Could you check a few things on this model? Use its own coordinates, in mm. A direction names the side the tool comes from. Round coordinates to 2 decimals unless told otherwise and drop trailing zeros. Write each loop counter-clockwise with the first axis right and the second up, starting at its lowest first coordinate (ties: lowest second). Pieces come first, ordered by that corner, then holes. Notation, with made-up numbers: (70, 83.5) -> (103, 83.5) arc R26 cw to (103, 105.5) -> close; hole circle Ø9 at (17, 41). An arc over 180 degrees is marked (long way). Return JSON: item names as keys, results as strings.
from build123d import *

# Parameters (mm, degrees)
EXTRUDE_1_DEPTH             = 20
CUT_EXTRUDE_1_DEPTH         = 15
EXTRUDE_2_DEPTH             = 15
HOLE_WIZARD_4_5_4_5_1_D     = 4.5
HOLE_WIZARD_4_5_4_5_1_DEPTH = 20
HOLE_WIZARD_20_0_20_1_D     = 20
HOLE_WIZARD_20_0_20_1_DEPTH = 20
HOLE_WIZARD_8_2_8_2_1_D     = 8.2
HOLE_WIZARD_8_2_8_2_1_DEPTH = 20
FILLET_1_R                  = 10


with BuildPart() as part:
    # 草图1 → 凸台-拉伸1 (new body)
    with BuildSketch(Plane(origin=(0, 0, 0), x_dir=(-1, 0, 0), z_dir=(0, 0, -1))):
        with BuildLine():
            ThreePointArc((-163.022889612, 198.274261736), (-150, 100), (-136.977110388, 198.274261736))
            ThreePointArc((-136.977110388, 198.274261736), (-140.459664046, 197.328853695), (-143.715646252, 195.773040012))
            ThreePointArc((-143.715646252, 195.773040012), (-144.596931613, 195.703918846), (-145.18869047, 196.36062508))
            ThreePointArc((-145.18869047, 196.36062508), (-150, 200), (-154.81130953, 196.36062508))
            ThreePointArc((-154.81130953, 196.36062508), (-155.403068387, 195.703918846), (-156.284353748, 195.773040012))
            ThreePointArc((-156.284353748, 195.773040012), (-159.540335954, 197.328853695), (-163.022889612, 198.274261736))
        make_face()
    extrude(amount=-EXTRUDE_1_DEPTH)

    # 草图2 → 切除-拉伸1 (cut)
    with BuildSketch(Plane.XY.offset(20)):
        with BuildLine():
            ThreePointArc((189.376148289, 164.838033327), (188.791059223, 165.557292987), (189.04835202, 166.448059))
            ThreePointArc((189.04835202, 166.448059), (189.837168574, 173), (183.768612947, 175.592835325))
            ThreePointArc((183.768612947, 175.592835325), (182.868540552, 175.815396233), (182.538187947, 176.681728058))
            ThreePointArc((182.538187947, 176.681728058), (169.336845119, 194.477731675), (150.795414997, 182.345602173))
            ThreePointArc((150.795414997, 182.345602173), (150.50949688, 181.851710417), (150, 181.594628396))
            ThreePointArc((150, 181.594628396), (149.49050312, 181.851710417), (149.204585003, 182.345602173))
            ThreePointArc((149.204585003, 182.345602173), (130.663154881, 194.477731675), (117.461812053, 176.681728058))
            ThreePointArc((117.461812053, 176.681728058), (117.131459448, 175.815396233), (116.231387053, 175.592835325))
            ThreePointArc((116.231387053, 175.592835325), (110.162831426, 173), (110.95164798, 166.448059))
            ThreePointArc((110.95164798, 166.448059), (111.208940777, 165.557292987), (110.623851711, 164.838033327))
            ThreePointArc((110.623851711, 164.838033327), (101.812731907, 144.507333265), (121.590179319, 134.516048507))
            ThreePointArc((121.590179319, 134.516048507), (122.160861185, 134.515382033), (122.638249186, 134.202685802))
            ThreePointArc((122.638249186, 134.202685802), (122.670358065, 133.63290755), (122.385594316, 133.138349319))
            ThreePointArc((122.385594316, 133.138349319), (121.149577026, 111.01493506), (143.162039659, 108.480238616))
            ThreePointArc((143.162039659, 108.480238616), (144.077481329, 108.62731078), (144.720260927, 107.959105675))
            ThreePointArc((144.720260927, 107.959105675), (150, 104), (155.279739073, 107.959105675))
            ThreePointArc((155.279739073, 107.959105675), (155.922518671, 108.62731078), (156.837960341, 108.480238616))
            ThreePointArc((156.837960341, 108.480238616), (178.850422974, 111.01493506), (177.614405684, 133.138349319))
            ThreePointArc((177.614405684, 133.138349319), (177.329641935, 133.63290755), (177.361750814, 134.202685802))
            ThreePointArc((177.361750814, 134.202685802), (177.839138815, 134.515382033), (178.409820681, 134.516048507))
            ThreePointArc((178.409820681, 134.516048507), (198.187268093, 144.507333265), (189.376148289, 164.838033327))
        make_face()
    extrude(amount=-CUT_EXTRUDE_1_DEPTH, mode=Mode.SUBTRACT)

    # 草图3 → 凸台-拉伸2 (add)
    with BuildSketch(Plane.XY.offset(5)):
        with BuildLine():
            ThreePointArc((150.795414997, 125.187925524), (150.50949688, 124.694033767), (150, 124.436951746))
            ThreePointArc((150, 124.436951746), (149.49050312, 124.694033767), (149.204585003, 125.187925524))
            ThreePointArc((149.204585003, 125.187925524), (141.575, 135.407471946), (128.909820681, 136.905113168))
            ThreePointArc((128.909820681, 136.905113168), (128.339138815, 136.905779642), (127.861750814, 137.218475873))
            ThreePointArc((127.861750814, 137.218475873), (127.829641935, 137.788254125), (128.114405684, 138.282812356))
            ThreePointArc((128.114405684, 138.282812356), (133.15, 150), (128.114405684, 161.717187644))
            ThreePointArc((128.114405684, 161.717187644), (127.829641935, 162.211745875), (127.861750814, 162.781524127))
            ThreePointArc((127.861750814, 162.781524127), (128.339138815, 163.094220358), (128.909820681, 163.094886832))
            ThreePointArc((128.909820681, 163.094886832), (141.575, 164.592528054), (149.204585003, 174.812074476))
            ThreePointArc((149.204585003, 174.812074476), (149.49050312, 175.305966233), (150, 175.563048254))
            ThreePointArc((150, 175.563048254), (150.50949688, 175.305966233), (150.795414997, 174.812074476))
            ThreePointArc((150.795414997, 174.812074476), (158.425, 164.592528054), (171.090179319, 163.094886832))
            ThreePointArc((171.090179319, 163.094886832), (171.660861185, 163.094220358), (172.138249186, 162.781524127))
            ThreePointArc((172.138249186, 162.781524127), (172.170358065, 162.211745875), (171.885594316, 161.717187644))
            ThreePointArc((171.885594316, 161.717187644), (166.85, 150), (171.885594316, 138.282812356))
            ThreePointArc((171.885594316, 138.282812356), (172.170358065, 137.788254125), (172.138249186, 137.218475873))
            ThreePointArc((172.138249186, 137.218475873), (171.660861185, 136.905779642), (171.090179319, 136.905113168))
            ThreePointArc((171.090179319, 136.905113168), (158.425, 135.407471946), (150.795414997, 125.187925524))
        make_face()
    extrude(amount=EXTRUDE_2_DEPTH)

    # Ø4.5 (4.5) 直径孔1
    with Locations(Plane(origin=(0, 0, 0), x_dir=(-1, 0, 0), z_dir=(0, 0, -1))):
        with Locations((-150, 195), (-111.02885683, 127.5), (-188.97114317, 127.5)):
            Hole(HOLE_WIZARD_4_5_4_5_1_D / 2, depth=HOLE_WIZARD_4_5_4_5_1_DEPTH)

    # Ø20.0 (20) 直径孔1
    with Locations(Plane(origin=(0, 0, 0), x_dir=(-1, 0, 0), z_dir=(0, 0, -1))):
        with Locations((-133.5, 178.578838325), (-117, 150), (-133.5, 121.421161675), (-166.5, 121.421161675), (-183, 150), (-166.5, 178.578838325)):
            Hole(HOLE_WIZARD_20_0_20_1_D / 2, depth=HOLE_WIZARD_20_0_20_1_DEPTH)

    # Ø8.2 (8.2) 直径孔1
    with Locations(Plane(origin=(0, 0, 0), x_dir=(-1, 0, 0), z_dir=(0, 0, -1))):
        with Locations((-114.925971147, 170.25), (-185.074028853, 170.25), (-150, 109.5)):
            Hole(HOLE_WIZARD_8_2_8_2_1_D / 2, depth=HOLE_WIZARD_8_2_8_2_1_DEPTH)

    # 圆角1
    fillet_1_edges = [part.edges().sort_by_distance(p)[0] for p in [
        (136.977110388, 198.274261736, 10),
        (163.022889612, 198.274261736, 10),
    ]]
    fillet(fillet_1_edges, radius=FILLET_1_R)


solid = part.part
1) I want a section at D-D, the plane x = 139.5. Count the separate pieces of the cut face and the enclosed holes in it, and give its area (3 significant figures).
Return value:
{"separate pieces": "3", "enclosed holes": "0", "area": "870 mm²"}
2) For faces 1 (the face through (151.97, 100.04, 9.86)), 2 (the face through (178.63, 110.76, 12.6)), 3 (the face through (157.68, 196.53, 9.86)), which set-ups out of +Z, -Z, +X, -X, +Y, -Y let a thin tool reach every point of the face, with its end or its side?
Return value:
{"face 1": "+Z, -Z", "face 2": "+Z", "face 3": "+Z, -Z, +Y"}
3) I want a section at A-A, the plane y = 154.5. Please give me the cut outline in (x, z).
Return value:
{"outline": "(100.2, 0) -> (108.07, 0) -> (108.07, 5) -> (101.49, 5) -> (101.49, 20) -> (100.2, 20) -> close; (125.93, 0) -> (174.07, 0) -> (174.07, 5) -> (167.49, 5) -> (167.49, 20) -> (132.51, 20) -> (132.51, 5) -> (125.93, 5) -> close; (191.93, 0) -> (199.8, 0) -> (199.8, 20) -> (198.51, 20) -> (198.51, 5) -> (191.93, 5) -> close"}
4) I want a section at C-C, the plane y = 190. Please give me the cut outline in (x, z).
Return value:
{"outline": "(120, 0) -> (180, 0) -> (180, 20) -> (177.92, 20) -> (177.92, 5) -> (155.08, 5) -> (155.08, 20) -> (144.92, 20) -> (144.92, 5) -> (122.08, 5) -> (122.08, 20) -> (120, 20) -> close"}
5) I want a section at B-B, the plane y = 127.5. Please give me the cut outline in (x, z).
Return value:
{"outline": "(105.35, 0) -> (108.78, 0) -> (108.78, 20) -> (105.35, 20) -> close; (113.28, 0) -> (125.56, 0) -> (125.56, 5) -> (118.54, 5) -> (118.54, 20) -> (113.28, 20) -> close; (141.44, 0) -> (158.56, 0) -> (158.56, 5) -> (151.54, 5) -> (151.54, 20) -> (148.46, 20) -> (148.46, 5) -> (141.44, 5) -> close; (174.44, 0) -> (186.72, 0) -> (186.72, 20) -> (181.46, 20) -> (181.46, 5) -> (174.44, 5) -> close; (191.22, 0) -> (194.65, 0) -> (194.65, 20) -> (191.22, 20) -> close"}
6) Will these pins go through, and if not, where does the flat tip stop? pin 1 Ø1 at (x, z) = (116.5, 4.5) entering from -Y; pin 2 Ø4 at (x, y) = (186.5, 162) entering from -Z; pin 3 Ø12 at (y, z) = (163, 9.5) entering from +X; pin 4 Ø4 at (x, y) = (188.97, 127.5) entering from -Z.
Return value:
{"pin 1": "y = 112.44", "pin 2": "z = 0", "pin 3": "x = 199.51", "pin 4": "through"}
7) Thinking about a two-plate mould opening in Y: for faces 4 (the face through (150, 184, 20)), 5 (the face through (117.13, 173.707, 2.535)), 6 (the face through (141.733, 135.315, 12.395)), 7 (the face through (142.28, 196.55, 9.86)), which applies, pulls with the +Y half, pulls with the -Y half, needs draft (parallel to the pull), parting line crosses it, or undercut?
Return value:
{"face 4": "needs draft", "face 5": "undercut", "face 6": "undercut", "face 7": "pulls with the +Y half"}
8) If I drill on probe 1 along X at (y, z) = (171, 4.5); probe 2 along Y at (x, z) = (189, 9); probe 3 along Y at (x, z) = (185, 1), over which ranges is the centre line in solid material (lowest first)? Write a range as [from, to].
Return value:
{"probe 1": "[104.62, 110.9], [118.96, 126.98], [140.02, 159.98], [173.02, 181.04], [189.1, 195.38]", "probe 2": "[118.71, 125.25], [129.75, 135.01], [165.12, 166.39], [174.1, 181.29]", "probe 3": "[114.29, 140.2], [159.8, 166.15], [174.35, 185.71]"}
